Design review of the part built by this model. Coordinates are the model's own, in mm. Give positions to 0.01 mm unless a question says otherwise; leave off trailing zeros. Write each loop counter-clockwise with the first axis right and the second up, starting at its lowest first coordinate (ties: lowest second). Pieces come first, ordered by that corner, then holes. Notation, with made-up numbers: (67.25, 48) - (101.25, 48) arc R22 cw to (101.25, 76) - close; hole circle Ø7 at (-37.75, 40.5). An arc over 180 degrees is marked (long way). Write each question's results on one line, items separated by ' | '. Start each with the question number.
from build123d import *

# Parameters (mm, degrees)
BOSS_EXTRUDE1_DEPTH = 90
SKETCH4_R           = 1.5
SKETCH4_R_2         = 4
CUT_EXTRUDE1_DEPTH  = 31
SKETCH6_R           = 4
SKETCH6_R_2         = 1.5
CUT_EXTRUDE2_DEPTH  = 31


with BuildPart() as part:
    # Sketch3 → Boss-Extrude1 (new body)
    with BuildSketch(Plane.XY):
        with BuildLine():
            Line((-2, 0.049393959), (-41, 0.049393959))
            Line((-41, 0.049393959), (-41, 2.049393959))
            Line((-41, 2.049393959), (-2.618272552, 2.049393959))
            ThreePointArc((-2.618272552, 2.049393959), (-2.194008483, 2.22512989), (-2.018272552, 2.649393959))
            Line((-2.018272552, 2.649393959), (-2.018272552, 26.449393959))
            ThreePointArc((-2.018272552, 26.449393959), (-2.194008483, 26.873658027), (-2.618272552, 27.049393959))
            Line((-2.618272552, 27.049393959), (-41.018189082, 27.049393959))
            Line((-41.018189082, 27.049393959), (-41.018189082, 29.049393959))
            Line((-41.018189082, 29.049393959), (-2.018189082, 29.049393959))
            ThreePointArc((-2.018189082, 29.049393959), (-0.60397552, 28.463607521), (-0.018189082, 27.049393959))
            Line((-0.018189082, 27.049393959), (-0.018189082, 2.049393959))
            ThreePointArc((-0.018189082, 2.049393959), (-0.597554333, 0.64159652), (-2, 0.049393959))
        make_face()
    extrude(amount=BOSS_EXTRUDE1_DEPTH)

    # Sketch4 → Cut-Extrude1 (cut)
    with BuildSketch(Plane(origin=(0, 29.049393959, 0), x_dir=(1, 0, 0), z_dir=(0, 1, 0))):
        with Locations(Location((-29.018189082, -3, 0), (0, 0, 180))):
            Circle(SKETCH4_R)
        with Locations(Location((-36.018189082, -10, 0), (0, 0, 180))):
            Circle(SKETCH4_R)
        with Locations(Location((-29.018189082, -10, 0), (0, 0, 180))):
            Circle(SKETCH4_R_2)
        with Locations(Location((-22.018189082, -10, 0), (0, 0, 180))):
            Circle(SKETCH4_R)
        with Locations(Location((-29.018189082, -17, 0), (0, 0, 180))):
            Circle(SKETCH4_R)
    extrude(amount=-CUT_EXTRUDE1_DEPTH, mode=Mode.SUBTRACT)

    # Sketch6 → Cut-Extrude2 (cut)
    with BuildSketch(Plane(origin=(0, 29.049393959, 0), x_dir=(1, 0, 0), z_dir=(0, 1, 0))):
        with Locations(Location((-29.018189082, -45.498892055, 0), (0, 0, 180))):
            Circle(SKETCH6_R)
        with Locations(Location((-29.018189082, -80.498892055, 0), (0, 0, 180))):
            Circle(SKETCH6_R)
        with Locations(Location((-36.018189082, -45.498892055, 0), (0, 0, 180))):
            Circle(SKETCH6_R_2)
        with Locations(Location((-36.018189082, -80.498892055, 0), (0, 0, 180))):
            Circle(SKETCH6_R_2)
        with Locations((5.981810918, -52.498892055)):
            Circle(SKETCH6_R_2)
        with Locations(Location((-29.018189082, -52.498892055, 0), (0, 0, 180))):
            Circle(SKETCH6_R_2)
        with Locations((-22.018189082, -10.498892055)):
            Circle(SKETCH6_R_2)
        with Locations(Location((-22.018189082, -45.498892055, 0), (0, 0, 180))):
            Circle(SKETCH6_R_2)
        with Locations((-64.018189082, -38.498892055)):
            Circle(SKETCH6_R_2)
        with Locations(Location((-29.018189082, -38.498892055, 0), (0, 0, 180))):
            Circle(SKETCH6_R_2)
        with Locations(Location((-29.018189082, -73.498892055, 0), (0, 0, 180))):
            Circle(SKETCH6_R_2)
        with Locations(Location((-22.018189082, -80.498892055, 0), (0, 0, 180))):
            Circle(SKETCH6_R_2)
        with Locations(Location((-29.018189082, -87.498892055, 0), (0, 0, 180))):
            Circle(SKETCH6_R_2)
    extrude(amount=-CUT_EXTRUDE2_DEPTH, mode=Mode.SUBTRACT)


solid = part.part
Q1. Add section D-D on y = 18. State the section outline as (x, z) points.
Q2. For line 1 along Y through (x, z) = (-35.5, 54); line 2 along X through (y, z) = (17.25, 69), list the stretches that pass through material, from the lowest coordinate up. Write a range as [from, to].
Q3. Insertion check: P1, Ø5, axis at x = -16.5, y = 22.5, coming from the -Z side; P2, Ø8, axis at y = 16.5, z = 37.5, coming from the -X side; P3, Ø4, axis at x = -29.02, z = 52.5, coming from the -Y side. Each pin has a flat end and moves straight along its axis. Give the tip position at first contact, or say it passes through.
Q4. Add section C-C on z = 57. State the section outline as (x, y) points, plus the area to 3 significant figures.
Q5. Add section B-B on x = -5.5. State the section outline as (y, z) points.
Q6. The part is to be moulded in two halves that separate along Z. For faces 1 (the face through (-22, 1, 12)), 2 (the face through (-18, 2.049, 44)), 3 (the face through (-22, 1, 47)), say which applies: +Z half, -Z half, draft (parallel to the pull), parting line (faces both ways), or undercut.
Q7. Add section A-A on z = 3. State the section outline as (x, y) points, plus the area to 3 significant figures.
Result:
1) outline: (-2.02, 0) - (-0.02, 0) - (-0.02, 90) - (-2.02, 90) - close
2) line 1: y = [0.05, 2.05], [27.05, 29.05] | line 2: x = [-2.02, -0.02]
3) P1: passes through | P2: stops at x = -2.02 | P3: stops at y = 0.05
4) outline: (-41.02, 27.05) - (-2.62, 27.05) arc R0.6 cw to (-2.02, 26.45) - (-2.02, 2.65) arc R0.6 cw to (-2.62, 2.05) - (-41, 2.05) - (-41, 0.05) - (-2, 0.05) arc R2 ccw to (-0.02, 2.05) - (-0.02, 27.05) arc R2 ccw to (-2.02, 29.05) - (-41.02, 29.05) - close | area: 212 mm²
5) outline: (0.05, 0) - (2.05, 0) - (2.05, 90) - (0.05, 90) - close; (27.05, 0) - (29.05, 0) - (29.05, 90) - (27.05, 90) - close
6) face 1: undercut | face 2: draft | face 3: undercut
7) outline: (-41.02, 27.05) - (-30.52, 27.05) - (-30.52, 29.05) - (-41.02, 29.05) - close; (-41, 0.05) - (-30.52, 0.05) - (-30.52, 2.05) - (-41, 2.05) - close; (-27.52, 0.05) - (-2, 0.05) arc R2 ccw to (-0.02, 2.05) - (-0.02, 27.05) arc R2 ccw to (-2.02, 29.05) - (-27.52, 29.05) - (-27.52, 27.05) - (-2.62, 27.05) arc R0.6 cw to (-2.02, 26.45) - (-2.02, 2.65) arc R0.6 cw to (-2.62, 2.05) - (-27.52, 2.05) - close | area: 200 mm²
